Part print with two shaded views. Sizes in mm from the minimum x, y, z corner. A direction names the side the tool comes from. Coordinates: 2 decimals unless noted, no trailing zeros. Loops run counter-clockwise (first coordinate to the right, second up) from the corner with the lowest first, then second, coordinate; pieces in that order, holes last. Notation, with made-up numbers: (-15.75, 60) -> (35.25, 60) arc R20 ccw to (35.25, 94) -> close; hole circle Ø7 at (86, 72). An arc over 180 degrees is marked (long way). Return JSON: item names as keys, results as strings. Group by question number.
(1) Tool access for the marked faces 4 and 5: list every direction of +Z, -Z, +X, -X, +Y, -Y with a clear straight run to the whole face (end or side of a thin tool).
(2) Saw through at B-B on z = 22. Write the cut outline in (x, y).
(3) Mould opens along Y. For the marked faces 1, 2 and 3 say: pulls with the +Y half, pulls with the -Y half, needs draft (parallel to the pull), parting line crosses it, or undercut.
(4) Saw through at C-C on x = 23. Write the cut outline in (y, z).
(5) Flat gauge pins, fed straight in: pin 1 Ø12 at (y, z) = (17, 20.5) entering from +X; pin 2 Ø9 at (y, z) = (25, 25) entering from -X; pin 3 Ø4 at (y, z) = (32.5, 17.5) entering from -X. Where does each tip first touch, or does it go through?
(6) Saw through at A-A on y = 25. Write the cut outline in (x, z).
(7) Probe L1, parallel to Y at x = 3.85, z = 25; L2, parallel to X at y = 41, z = 19. List the from-to ranges inside material, lowest first.
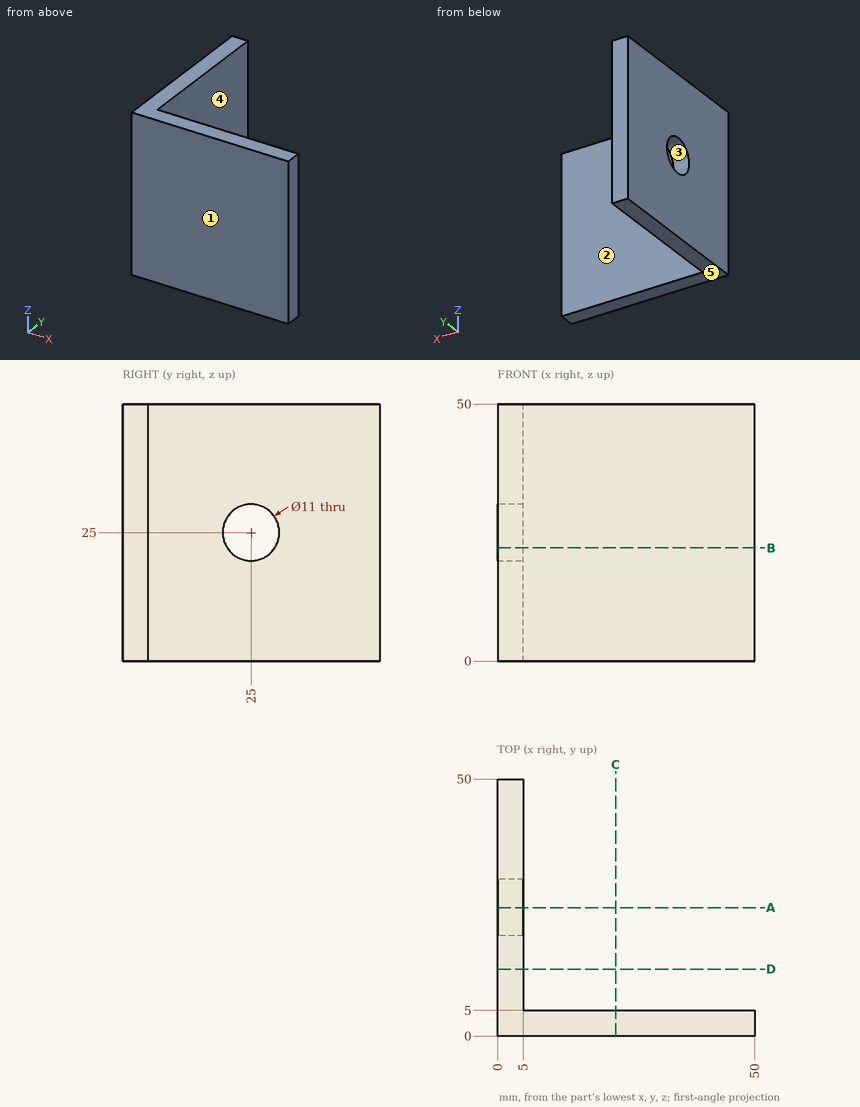
Geometry results:
{
 "1": {"face 4": "+Z, -Z, +X, +Y", "face 5": "-Z, +X, -X, +Y, -Y"},
 "2": {"outline": "(0, 0) -> (50, 0) -> (50, 5) -> (5, 5) -> (5, 20.39) -> (0, 20.39) -> close; (0, 29.61) -> (5, 29.61) -> (5, 50) -> (0, 50) -> close"},
 "3": {"face 1": "pulls with the -Y half", "face 2": "pulls with the +Y half", "face 3": "undercut"},
 "4": {"outline": "(0, 0) -> (5, 0) -> (5, 50) -> (0, 50) -> close"},
 "5": {"pin 1": "x = 5", "pin 2": "through", "pin 3": "x = 0"},
 "6": {"outline": "(0, 0) -> (5, 0) -> (5, 19.5) -> (0, 19.5) -> close; (0, 30.5) -> (5, 30.5) -> (5, 50) -> (0, 50) -> close"},
 "7": {"L1": "0 to 19.5, 30.5 to 50", "L2": "0 to 5"}
}
